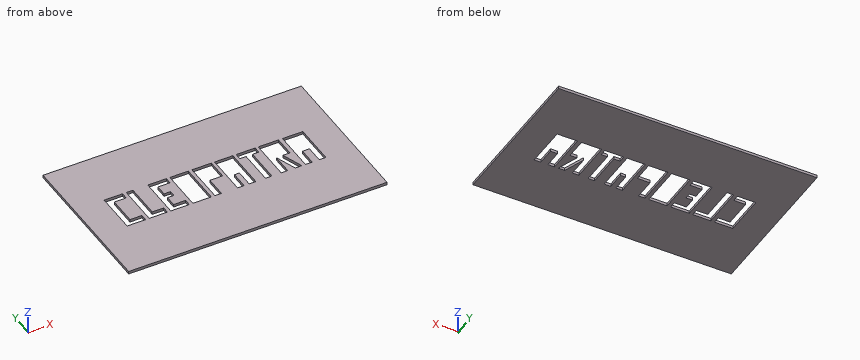
from build123d import *

# Parameters (mm, degrees)
SKETCH1_W           = 297.18
SKETCH1_H           = 177.8
BOSS_EXTRUDE1_DEPTH = 3.175
SKETCH3_W           = 13.69262242
SKETCH3_H           = 7.623435988
SKETCH3_W_2         = 7.48484453
SKETCH3_H_2         = 16.262538767
SKETCH3_H_3         = 16.21355287
SKETCH3_H_4         = 7.672421885
SKETCH3_W_3         = 7.714624958
SKETCH3_H_5         = 23.885974755
SKETCH3_W_4         = 13.165983096
SKETCH3_W_5         = 7.502078631
SKETCH3_H_6         = 3.540074356
SKETCH3_W_6         = 7.385030665
SKETCH3_H_7         = 12.673478514
SKETCH3_W_7         = 13.868168861
SKETCH3_H_8         = 12.722464411
SKETCH3_W_8         = 7.610546603
SKETCH3_H_9         = 8.377243284
SKETCH3_H_10        = 7.522942085
SKETCH3_W_9         = 7.199942392
SKETCH3_W_10        = 7.545958675
SKETCH3_H_11        = 0.313367501
SKETCH3_W_11        = 6.151941086
SKETCH3_W_12        = 7.563125845
SKETCH3_W_13        = 5.793032563
SKETCH3_W_14        = 7.724043416
SKETCH3_H_12        = 12.138714327
SKETCH3_H_13        = 20.136219216
SKETCH3_H_14        = 4.074838543
SKETCH3_H_15        = 3.749755539
SKETCH3_W_15        = 7.197404092
SKETCH3_W_16        = 7.446094885
SKETCH3_W_17        = 7.592383586
SKETCH3_W_18        = 8.426229181
SKETCH3_W_19        = 7.372950534
SKETCH3_H_16        = 7.836309586
SKETCH3_W_20        = 7.738672287
SKETCH3_W_21        = 8.057581655
SKETCH3_W_22        = 7.668237515
CUT_EXTRUDE4_DEPTH  = 3.175


with BuildPart() as part:
    # Sketch1 → Boss-Extrude1 (new body)
    with BuildSketch(Plane.XY):
        Rectangle(SKETCH1_W, SKETCH1_H)
    extrude(amount=BOSS_EXTRUDE1_DEPTH)

    # Sketch3 → Cut-Extrude4 (cut)
    with BuildSketch(Plane.XY.offset(3.175)):
        with Locations((-99.96884426, 20.074256761)):
            Rectangle(SKETCH3_W, SKETCH3_H)
        with Locations((-110.557577735, 20.074256761)):
            Rectangle(SKETCH3_W_2, SKETCH3_H)
        with Locations((-110.557577735, 8.131269384)):
            Rectangle(SKETCH3_W_2, SKETCH3_H_2)
        with Locations((-110.557577735, -8.106776435)):
            Rectangle(SKETCH3_W_2, SKETCH3_H_3)
        with Locations((-110.557577735, -20.049763813)):
            Rectangle(SKETCH3_W_2, SKETCH3_H_4)
        with Locations((-99.96884426, -20.049763813)):
            Rectangle(SKETCH3_W, SKETCH3_H_4)
        with Locations((-85.042687521, 11.942987378)):
            Rectangle(SKETCH3_W_3, SKETCH3_H_5)
        with Locations((-85.042687521, -8.106776435)):
            Rectangle(SKETCH3_W_3, SKETCH3_H_3)
        with Locations((-74.602383494, -20.049763813)):
            Rectangle(SKETCH3_W_4, SKETCH3_H_4)
        with Locations((-85.042687521, -20.049763813)):
            Rectangle(SKETCH3_W_3, SKETCH3_H_4)
        with Locations((-60.359912579, 1.770037178)):
            Rectangle(SKETCH3_W_5, SKETCH3_H_6)
        with Locations((-52.916357931, 1.770037178)):
            Rectangle(SKETCH3_W_6, SKETCH3_H_6)
        with Locations((-52.916357931, -1.770037178)):
            Rectangle(SKETCH3_W_6, SKETCH3_H_6)
        with Locations((-60.359912579, -1.770037178)):
            Rectangle(SKETCH3_W_5, SKETCH3_H_6)
        with Locations((-60.359912579, -9.876813613)):
            Rectangle(SKETCH3_W_5, SKETCH3_H_7)
        with Locations((-60.359912579, -20.049763813)):
            Rectangle(SKETCH3_W_5, SKETCH3_H_4)
        with Locations((-49.674788833, -20.049763813)):
            Rectangle(SKETCH3_W_7, SKETCH3_H_4)
        with Locations((-60.359912579, 9.901306562)):
            Rectangle(SKETCH3_W_5, SKETCH3_H_8)
        with Locations((-60.359912579, 20.074256761)):
            Rectangle(SKETCH3_W_5, SKETCH3_H)
        with Locations((-49.674788833, 20.074256761)):
            Rectangle(SKETCH3_W_7, SKETCH3_H)
        Polygon((-25.010513832, 0), (-17.462016857, 0), (-17.462016857, 23.885974755), (-38.710951894, 23.885974755), (-38.710951894, 0), (-31.162454918, 0), (-31.162454918, 16.21355287), (-25.010513832, 16.21355287), align=None)
        Polygon((-17.462016857, -23.885974755), (-17.462016857, 0), (-25.010513832, 0), (-25.010513832, -16.21355287), (-31.162454918, -16.21355287), (-31.162454918, 0), (-38.710951894, 0), (-38.710951894, -23.885974755), align=None)
        with Locations((-9.505678593, -11.942987378)):
            Rectangle(SKETCH3_W_8, SKETCH3_H_5)
        with Locations((-9.505678593, 20.049763813)):
            Rectangle(SKETCH3_W_8, SKETCH3_H_4)
        with Locations((-9.505678593, 12.024931228)):
            Rectangle(SKETCH3_W_8, SKETCH3_H_9)
        with Locations((-9.505678593, 4.074838544)):
            Rectangle(SKETCH3_W_8, SKETCH3_H_10)
        with Locations((-2.100434095, 4.074838544)):
            Rectangle(SKETCH3_W_9, SKETCH3_H_10)
        with Locations((5.272516439, 4.074838544)):
            Rectangle(SKETCH3_W_10, SKETCH3_H_10)
        with Locations((5.272516439, 12.024931228)):
            Rectangle(SKETCH3_W_10, SKETCH3_H_9)
        with Locations((5.272516439, 20.049763813)):
            Rectangle(SKETCH3_W_10, SKETCH3_H_4)
        with Locations((-2.100434095, 20.049763813)):
            Rectangle(SKETCH3_W_9, SKETCH3_H_4)
        with Locations((-9.505678593, 0.15668375)):
            Rectangle(SKETCH3_W_8, SKETCH3_H_11)
        with Locations((-28.086484375, 8.106776435)):
            Rectangle(SKETCH3_W_11, SKETCH3_H_3)
        with Locations((-28.086484375, -8.106776435)):
            Rectangle(SKETCH3_W_11, SKETCH3_H_3)
        with Locations((-2.100434095, 12.024931228)):
            Rectangle(SKETCH3_W_9, SKETCH3_H_9)
        with Locations((16.498905095, 20.049763813)):
            Rectangle(SKETCH3_W_12, SKETCH3_H_4)
        with Locations((23.176984299, 20.049763813)):
            Rectangle(SKETCH3_W_13, SKETCH3_H_4)
        with Locations((29.935522289, 20.049763813)):
            Rectangle(SKETCH3_W_14, SKETCH3_H_4)
        with Locations((29.935522289, 10.144195706)):
            Rectangle(SKETCH3_W_14, SKETCH3_H_12)
        with Locations((16.498905095, 10.144195706)):
            Rectangle(SKETCH3_W_12, SKETCH3_H_12)
        with Locations((16.498905095, -13.817865147)):
            Rectangle(SKETCH3_W_12, SKETCH3_H_13)
        with Locations((29.935522289, -13.817865147)):
            Rectangle(SKETCH3_W_14, SKETCH3_H_13)
        with Locations((23.176984299, 2.037419272)):
            Rectangle(SKETCH3_W_13, SKETCH3_H_14)
        with Locations((23.176984299, -1.87487777)):
            Rectangle(SKETCH3_W_13, SKETCH3_H_15)
        with Locations((16.498905095, -1.87487777)):
            Rectangle(SKETCH3_W_12, SKETCH3_H_15)
        with Locations((16.498905095, 2.037419272)):
            Rectangle(SKETCH3_W_12, SKETCH3_H_14)
        with Locations((29.935522289, 2.037419272)):
            Rectangle(SKETCH3_W_14, SKETCH3_H_14)
        with Locations((29.935522289, -1.87487777)):
            Rectangle(SKETCH3_W_14, SKETCH3_H_15)
        with Locations((23.176984299, 10.144195706)):
            Rectangle(SKETCH3_W_13, SKETCH3_H_12)
        with Locations((41.185123401, 20.049763813)):
            Rectangle(SKETCH3_W_15, SKETCH3_H_4)
        with Locations((48.50687289, 20.049763813)):
            Rectangle(SKETCH3_W_16, SKETCH3_H_4)
        with Locations((55.828622378, 20.049763813)):
            Rectangle(SKETCH3_W_15, SKETCH3_H_4)
        with Locations((48.50687289, 8.106776435)):
            Rectangle(SKETCH3_W_16, SKETCH3_H_3)
        with Locations((66.690558432, 20.049763813)):
            Rectangle(SKETCH3_W_17, SKETCH3_H_4)
        with Locations((74.699864816, 20.049763813)):
            Rectangle(SKETCH3_W_18, SKETCH3_H_4)
        with Locations((48.50687289, -11.942987378)):
            Rectangle(SKETCH3_W_16, SKETCH3_H_5)
        with Locations((82.599454673, 20.049763813)):
            Rectangle(SKETCH3_W_19, SKETCH3_H_4)
        with Locations((74.699864816, 12.024931228)):
            Rectangle(SKETCH3_W_18, SKETCH3_H_9)
        with Locations((66.690558432, 12.024931228)):
            Rectangle(SKETCH3_W_17, SKETCH3_H_9)
        with Locations((82.599454673, 12.024931228)):
            Rectangle(SKETCH3_W_19, SKETCH3_H_9)
        Polygon((70.486750225, 7.836309586), (70.486750225, 0), (78.106750225, 0), (86.28592994, 0), (86.28592994, 7.836309586), (78.912979406, 7.836309586), align=None)
        Polygon((78.106750225, 0), (70.486750225, 0), (79.088525848, -23.885974755), (86.708525848, -23.885974755), align=None)
        with Locations((66.690558432, -11.942987378)):
            Rectangle(SKETCH3_W_17, SKETCH3_H_5)
        with Locations((66.690558432, 3.918154793)):
            Rectangle(SKETCH3_W_17, SKETCH3_H_16)
        with Locations((94.704844686, 20.049763813)):
            Rectangle(SKETCH3_W_20, SKETCH3_H_4)
        with Locations((102.602971658, 20.049763813)):
            Rectangle(SKETCH3_W_21, SKETCH3_H_4)
        with Locations((94.704844686, 10.144195706)):
            Rectangle(SKETCH3_W_20, SKETCH3_H_12)
        with Locations((110.465881243, 20.049763813)):
            Rectangle(SKETCH3_W_22, SKETCH3_H_4)
        with Locations((110.465881243, 10.144195706)):
            Rectangle(SKETCH3_W_22, SKETCH3_H_12)
        with Locations((110.465881243, -13.817865147)):
            Rectangle(SKETCH3_W_22, SKETCH3_H_13)
        with Locations((102.602971658, 10.144195706)):
            Rectangle(SKETCH3_W_21, SKETCH3_H_12)
        with Locations((94.704844686, -1.87487777)):
            Rectangle(SKETCH3_W_20, SKETCH3_H_15)
        with Locations((94.704844686, 2.037419272)):
            Rectangle(SKETCH3_W_20, SKETCH3_H_14)
        with Locations((110.465881243, 2.037419272)):
            Rectangle(SKETCH3_W_22, SKETCH3_H_14)
        with Locations((102.602971658, -1.87487777)):
            Rectangle(SKETCH3_W_21, SKETCH3_H_15)
        with Locations((94.704844686, -13.817865147)):
            Rectangle(SKETCH3_W_20, SKETCH3_H_13)
        with Locations((102.602971658, 2.037419272)):
            Rectangle(SKETCH3_W_21, SKETCH3_H_14)
        with Locations((110.465881243, -1.87487777)):
            Rectangle(SKETCH3_W_22, SKETCH3_H_15)
    extrude(amount=-CUT_EXTRUDE4_DEPTH, mode=Mode.SUBTRACT)


solid = part.part
Geometry check sheet. Reference: the model listing, model coordinates, mm. Give positions to 0.01 mm unless a question says otherwise; leave off trailing zeros. Loops run counter-clockwise (first coordinate to the right, second up) from the corner with the lowest first, then second, coordinate; pieces in that order, holes last. Notation, with made-up numbers: M -20,-0.75 L 14,-0.75 A9 ccw 14,4.25 Z; hole C 21,52.25 d8. An arc over 180 degrees is marked long. Answer as a JSON object with one key per item and string values. Group by question number.
Item 1: Material ranges on L1, parallel to Y at x = -77, z = 3; L2, parallel to Y at x = 67.5, z = 2.85, recorded low to high.
Item 2: Sectioned sample at B-B on x = 103. Record the boundary of the cut face in (y, z) (3 decimals), plus the area to 3 significant figures.
Item 3: Sectioned sample at C-C on z = 2.6. Give the number of separate pieces and of enclosed holes in the cut face, plus the area to 3 significant figures.
Item 4: Sectioned sample at A-A on x = -23.5. Record the boundary of the cut face in (y, z) (3 decimals), plus the area to 3 significant figures.
Findings below:
{
 "1": {"L1": "-88.9 to -23.89, -16.21 to 88.9", "L2": "-88.9 to -23.89, 23.89 to 88.9"},
 "2": {"outline": "M -88.9,0 L -3.75,0 L -3.75,3.175 L -88.9,3.175 Z; M 23.886,0 L 88.9,0 L 88.9,3.175 L 23.886,3.175 Z", "area": "477 mm2"},
 "3": {"separate pieces": "1", "enclosed holes": "9", "area": "46,200 mm2"},
 "4": {"outline": "M -88.9,0 L -23.886,0 L -23.886,3.175 L -88.9,3.175 Z; M 23.886,0 L 88.9,0 L 88.9,3.175 L 23.886,3.175 Z", "area": "413 mm2"}
}
